Can you work these out from the model? Positions are in its coordinate system, mm. Give positions to 0.01 mm unless a question says otherwise; leave off trailing zeros. Order: outer loops, then holes, each group sorted by start corner. A loop starts at its lowest first (then second) coordinate and runs counter-clockwise, first axis right, second up. Notation, with made-up numbers: (87, -23.5) - (143, -23.5) arc R18 ccw to (143, -1.5) - close; hole circle Ø9 at (7.25, -12.75). An arc over 180 degrees is marked (long way). One line per question, with ' | ' between items.
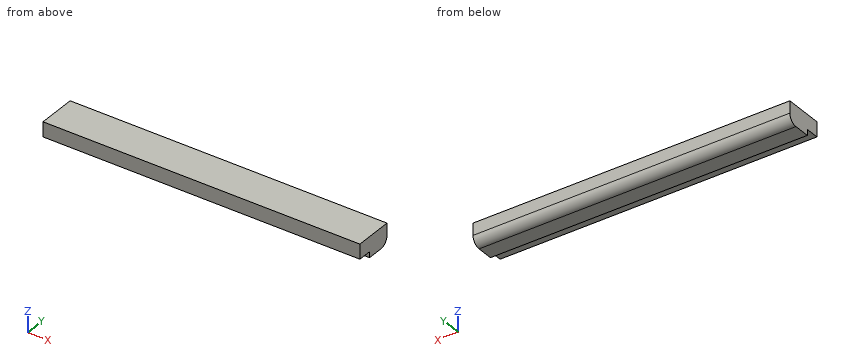
```python
from build123d import *

# Parameters (mm, degrees)
ESQUISSE1_W             = 462
ESQUISSE1_H             = 56
BOSS_EXTRU_1_DEPTH      = 21.5
BOSS_EXTRU_1_DEPTH_BACK = 8.5
ENL_V_START             = -8.5
ESQUISSE2_W             = 462
ESQUISSE2_H             = 20
ENL_V_MAT_EXTRU_2_DEPTH = 8.5
CONG_1_R                = 12.5


with BuildPart() as part:
    # Esquisse1 → Boss.-Extru.1 (new body, two sides)
    with BuildSketch(Plane.XY) as boss_extru_1_sk:
        with Locations((30, 8)):
            Rectangle(ESQUISSE1_W, ESQUISSE1_H)
    extrude(amount=BOSS_EXTRU_1_DEPTH)
    extrude(boss_extru_1_sk.sketch, amount=-BOSS_EXTRU_1_DEPTH_BACK)

    # Esquisse2 → Enl_v. mat.-Extru.2 (cut)
    with BuildSketch(Plane(origin=(0, 0, -8.5), x_dir=(-1, 0, 0), z_dir=(0, 0, -1)).offset(ENL_V_START)):
        with Locations((-30, -10)):
            Rectangle(ESQUISSE2_W, ESQUISSE2_H)
    extrude(amount=ENL_V_MAT_EXTRU_2_DEPTH, mode=Mode.SUBTRACT)

    # Cong_1
    cong_1_edges = [part.edges().sort_by_distance(p)[0] for p in [
        (30, 36, -8.5),
    ]]
    fillet(cong_1_edges, radius=CONG_1_R)


solid = part.part
```
(1) Imagine slicing it at B-B (y = -9). List the corners of the cut face in (x, z) for me.
Answer below:
outline: (-201, 0) - (261, 0) - (261, 21.5) - (-201, 21.5) - close
(2) Will these pins go through, and if not, where does the flat tip stop? pin 1 (3 mm diameter, centred on x = -6.5, z = -4, fed in from +Y); pin 2 (16 mm diameter, centred on x = -78, y = -8.5, fed in from -Z).
Answer below:
pin 1: y = 34.18 | pin 2: z = 0
(3) Imagine slicing it at A-A (x = -142.5). List the corners of the cut face in (y, z) for me, and give its area (3 significant figures).
Answer below:
outline: (-20, 0) - (0, 0) - (0, -8.5) - (23.5, -8.5) arc R12.5 ccw to (36, 4) - (36, 21.5) - (-20, 21.5) - close | area: 1,480 mm^2
(4) If I drill on line 1 (Z direction, x = -106.5, y = -9); line 2 (Z direction, x = 185, y = 25); line 3 (Y direction, x = 13, z = -2.5), over which ranges is the centre line in solid material (lowest first)?
Answer below:
line 1: 0 to 21.5 | line 2: -8.41 to 21.5 | line 3: 0 to 34.18
